Source: CAD feature listing. Evaluate the final solid. Frame: model axes, mm. A direction names the side the tool comes from. Coordinates: 2 decimals unless noted, no trailing zeros. Loops run counter-clockwise (first coordinate to the right, second up) from the corner with the lowest first, then second, coordinate; pieces in that order, holes last.
Item 1: Pin query (flat end, axial travel): pin 1 Ø5 at (x, z) = (173.5, -101) entering from -Y; pin 2 Ø4 at (y, z) = (7, -105.5) entering from -X; pin 3 Ø1 at (x, y) = (-9.5, 7.5) entering from +Z. Return the tip coordinate at first contact, or that it passes through.
Item 2: Pull-direction query (Z, two-part tool) for faces 1 (the flat face through (95, 0, -61)), 2 (the cylindrical face through (-62.594, 5.07, -90.219)), 3 (the cylindrical face through (247.719, 5.07, -2.406)); classes: +Z half, -Z half, draft (parallel to the pull), parting line (faces both ways), or undercut.
Item 3: Line query: probe 1 along Z at (x, y) = (-39, 8.5); probe 2 along X at (y, z) = (0.75, -22); probe 3 along Z at (x, y) = (-14, 0.5). Output: solid intervals per line, ascending.
Item 4: Section query B-B, the plane z = -102. Return the cut outline in (x, y), then the cut area to 3 significant figures.
Item 5: Reachability of faces 4 (the flat face through (-43, 5, -27.5)), 5 (the flat face through (95, 10, -61)), 6 (the flat face through (-44, 5, -92.5)) from +Z, -Z, +X, -X, +Y, -Y: full face, straight path, thin tool, end or side. Return the list, or none.
Item 6: Section query A-A, the plane y = 5. Return the cut outline in (x, z), then the cut area to 3 significant figures.
```python
from build123d import *

# Parameters (mm, degrees)
BOSS_EXTRUDE1_DEPTH = 10
FILLET1_R           = 8


with BuildPart() as part:
    # Sketch1 → Boss-Extrude1 (new body)
    with BuildSketch(Plane(origin=(0, 0, 0), x_dir=(1, 0, 0), z_dir=(0, 1, 0))):
        with BuildLine():
            Line((-65, 92.5), (-30, 92.5))
            ThreePointArc((-30, 92.5), (-9.651474255, 100.415244642), (0, 120))
            Line((0, 120), (250, 120))
            Line((250, 120), (250, 0))
            Line((250, 0), (0, 0))
            ThreePointArc((0, 0), (-9.651474255, 19.584755358), (-30, 27.5))
            Line((-30, 27.5), (-65, 27.5))
            Line((-65, 27.5), (-65, 92.5))
        make_face()
    extrude(amount=BOSS_EXTRUDE1_DEPTH)

    # Fillet1
    fillet1_edges = [part.edges().sort_by_distance(p)[0] for p in [
        (-65, 5, -92.5),
        (0, 5, -120),
        (250, 5, -120),
        (250, 5, 0),
        (0, 5, 0),
        (-65, 5, -27.5),
    ]]
    fillet(fillet1_edges, radius=FILLET1_R)


solid = part.part
```
Verdict:
1. pin 1: stops at y = 0
1. pin 2: stops at x = -6.73
1. pin 3: stops at z = -18.97
2. face 1: draft
2. face 2: -Z half
2. face 3: +Z half
3. probe 1: z = -92.5 to -27.5
3. probe 2: x = -12.65 to 250
3. probe 3: z = -97.1 to -22.9
4. outline: (-8.05, 0) - (250, 0) - (250, 10) - (-8.05, 10) - close
4. area: 2,580 mm2
5. face 4: +Z, -X, +Y, -Y
5. face 5: +Z, -Z, +X, -X, +Y
5. face 6: -Z, -X, +Y, -Y
6. outline: (-65, -84.5) arc R8 ccw to (-57, -92.5) - (-30, -92.5) arc R30.11 cw to (-1.08, -114.23) arc R8 ccw to (6.61, -120) - (242, -120) arc R8 ccw to (250, -112) - (250, -8) arc R8 ccw to (242, 0) - (6.61, 0) arc R8 ccw to (-1.08, -5.77) arc R30.11 cw to (-30, -27.5) - (-57, -27.5) arc R8 ccw to (-65, -35.5) - close
6. area: 34,500 mm2
